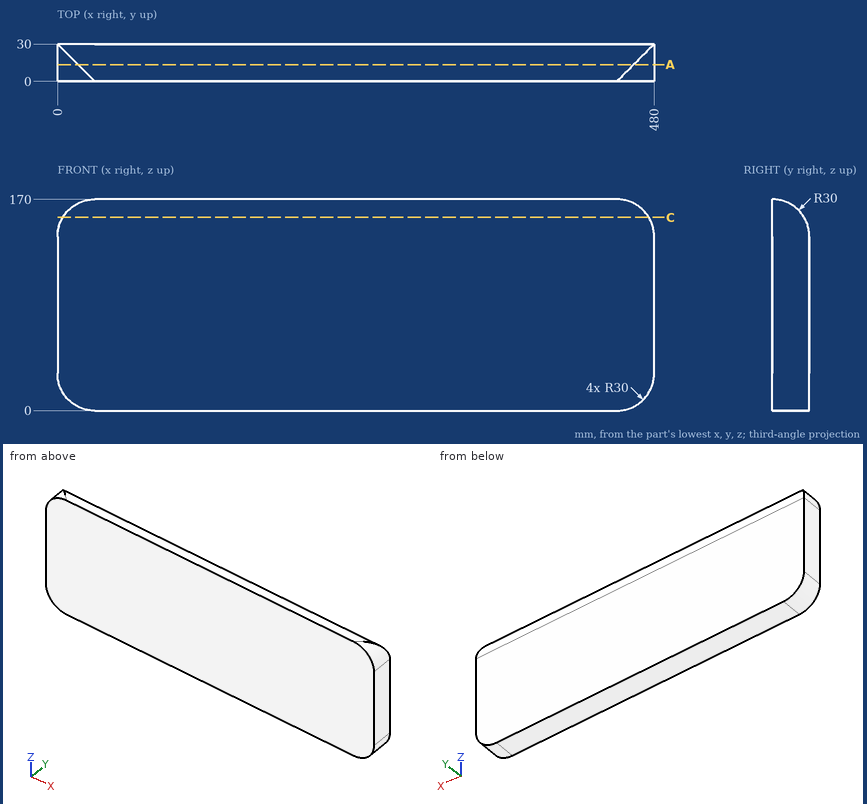
Design review of the part shown in the three views and the two pictorial views. Dimensions are in mm from the part's minimum x, y and z. Coordinates: 2 decimals unless noted, no trailing zeros. Loops run counter-clockwise (first coordinate to the right, second up) from the corner with the lowest first, then second, coordinate; pieces in that order, holes last.
(1) Wall thickness on L1, parallel to X at y = 13.5, z = 29; L2, parallel to Z at x = 122, y = 12 (1 decimal); L3, parallel to Z at x = 63.5, y = 20: over which ranges is each line inside the solid? List them lowest first.
Determined:
L1: x = 0.02 to 479.98
L2: z = 0 to 167.5
L3: z = 0 to 162.36
(2) Consider section A-A, the plane y = 13.5. Give the boundary of the cut face in (x, z), plus the area to 3 significant figures.
Determined:
outline: (0, 30) arc R30 ccw to (30, 0) - (450, 0) arc R30 ccw to (480, 30) - (480, 140) arc R30 ccw to (463.5, 166.79) - (16.5, 166.79) arc R30 ccw to (0, 140) - close
area: 79,400 mm2
(3) Insertion check: P1, Ø1, axis at x = 189, y = 23.5, coming from the +Z side; P2, Ø4, axis at x = 192.5, y = 26.5, coming from the +Z side (1 decimal); P3, Ø12, axis at x = 157, y = 7.5, coming from the +Z side. Each pin has a flat end and moves straight along its axis. Give the tip position at first contact, or say it passes through.
Determined:
P1: stops at z = 159.26
P2: stops at z = 157.3
P3: stops at z = 169.96
(4) Consider section C-C, the plane z = 155.5. Give the boundary of the cut face in (x, y) (1 decimal).
Determined:
outline: (4.3, 0) - (475.7, 0) - (475.7, 25.7) - (4.3, 25.7) - close
